Source: CAD feature listing. Evaluate the final solid. Frame: model axes, mm. A direction names the side the tool comes from. Round coordinates to 2 decimals unless told otherwise and drop trailing zeros. Write each loop counter-clockwise with the first axis right and the second up, starting at its lowest first coordinate (ties: lowest second). Pieces come first, ordered by that corner, then holes. Notation, with made-up numbers: (-35.5, 26) -> (-16.5, 26) arc R20 cw to (-16.5, 40) -> close; hole circle Ø6 at (-12.5, -14). An arc over 180 degrees is marked (long way). Put each result on its own line as item: value.
```python
from build123d import *

# Parameters (mm, degrees)
SKETCH1_R           = 1.5
BOSS_EXTRUDE1_DEPTH = 4
SKETCH2_W           = 24
SKETCH2_H           = 4
CUT_EXTRUDE1_DEPTH  = 10


with BuildPart() as part:
    # Sketch1 → Boss-Extrude1 (new body)
    with BuildSketch(Plane.XY):
        with BuildLine():
            Line((25.5, -2), (7.5, -2))
            ThreePointArc((7.5, -2), (6.085786438, -1.414213562), (5.5, 0))
            ThreePointArc((5.5, 0), (-0.650170894, 5.461435508), (-5.34628284, -1.291224148))
            ThreePointArc((-5.34628284, -1.291224148), (-4.25, -10.5), (-5.34628284, -19.708775852))
            ThreePointArc((-5.34628284, -19.708775852), (1.057902641, -26.39729951), (4.463242224, -17.786050895))
            ThreePointArc((4.463242224, -17.786050895), (3.8789457, -10.047752676), (10.5, -6))
            Line((10.5, -6), (25.5, -6))
            Line((25.5, -6), (25.5, -2))
        make_face()
        Circle(SKETCH1_R, mode=Mode.SUBTRACT)
        with Locations((0, -21)):
            Circle(SKETCH1_R, mode=Mode.SUBTRACT)
    extrude(amount=BOSS_EXTRUDE1_DEPTH)

    # Sketch2 → Cut-Extrude1 (cut)
    with BuildSketch(Plane.XY.offset(4)):
        with Locations((13.5, -8)):
            Rectangle(SKETCH2_W, SKETCH2_H)
    extrude(amount=-CUT_EXTRUDE1_DEPTH, mode=Mode.SUBTRACT)


solid = part.part
```
Q1. Cut plane B-B on x = 0. Output: boundary loops of the cut face in (y, z), and give its area (3 significant figures).
Ans:
outline: (-26.5, 0) -> (-22.5, 0) -> (-22.5, 4) -> (-26.5, 4) -> close; (-19.5, 0) -> (-1.5, 0) -> (-1.5, 4) -> (-19.5, 4) -> close; (1.5, 0) -> (5.5, 0) -> (5.5, 4) -> (1.5, 4) -> close
area: 104 mm^2
Q2. Reachability of faces 1 (the cylindrical face through (0.906, -26.425, 1.972)), 2 (the flat face through (3, -10, 2)) from +Z, -Z, +X, -X, +Y, -Y: full face, straight path, thin tool, end or side. Return the list, or none.
Ans:
face 1: +Z, -Z
face 2: +Z, -Z, +X
Q3. Draft query along Y for faces 3 (the cylindrical face through (-0.195, -19.513, 1.972)), 4 (the cylindrical face through (3.084, -14.03, 1.972)), 5 (the flat face through (17, -2, 2)), 6 (the flat face through (4.2, -5.7, 0)). Return one class per face: +Y half, -Y half, draft (parallel to the pull), parting line (faces both ways), or undercut.
Ans:
face 3: undercut
face 4: undercut
face 5: +Y half
face 6: draft
Q4. Cut plane A-A on y = -21. Output: boundary loops of the cut face in (x, z).
Ans:
outline: (-5.5, 0) -> (-1.5, 0) -> (-1.5, 4) -> (-5.5, 4) -> close; (1.5, 0) -> (5.5, 0) -> (5.5, 4) -> (1.5, 4) -> close
Q5. Material intervals for line 1 (Y direction, x = 0, z = 2.8); line 2 (Y direction, x = 15.5, z = 3.7); line 3 (X direction, y = -0.5, z = 2.55), sorted ascending. Write a range as [from, to].
Ans:
line 1: y = [-26.5, -22.5], [-19.5, -1.5], [1.5, 5.5]
line 2: y = [-6, -2]
line 3: x = [-5.48, -1.41], [1.41, 5.56]
Q6. Cut plane C-C on z = 3. Output: boundary loops of the cut face in (x, y) (3 decimals), and give its area (3 significant figures).
Ans:
outline: (-5.346, -19.709) arc R5.5 ccw (long way) to (4.463, -17.786) arc R7.439 cw to (3.904, -10) -> (1.5, -10) -> (1.5, -6) -> (25.5, -6) -> (25.5, -2) -> (7.5, -2) arc R2 cw to (5.5, 0) arc R5.5 ccw (long way) to (-5.346, -1.291) arc R39.225 cw to start; hole circle Ø3 at (0, -21); hole circle Ø3 at (0, 0)
area: 343 mm^2
Q7. Pin query (flat end, axial travel): pin 1 (0.7 mm diameter, centred on x = 2, z = 2.5, fed in from +Y); pin 2 (2 mm diameter, centred on x = 17.5, z = 2, fed in from -Y). Return the tip coordinate at first contact, or that it passes through.
Ans:
pin 1: stops at y = 5.25
pin 2: stops at y = -6
Q8. Cut plane D-D on x = 11.5. Output: boundary loops of the cut face in (y, z).
Ans:
outline: (-6, 0) -> (-2, 0) -> (-2, 4) -> (-6, 4) -> close
